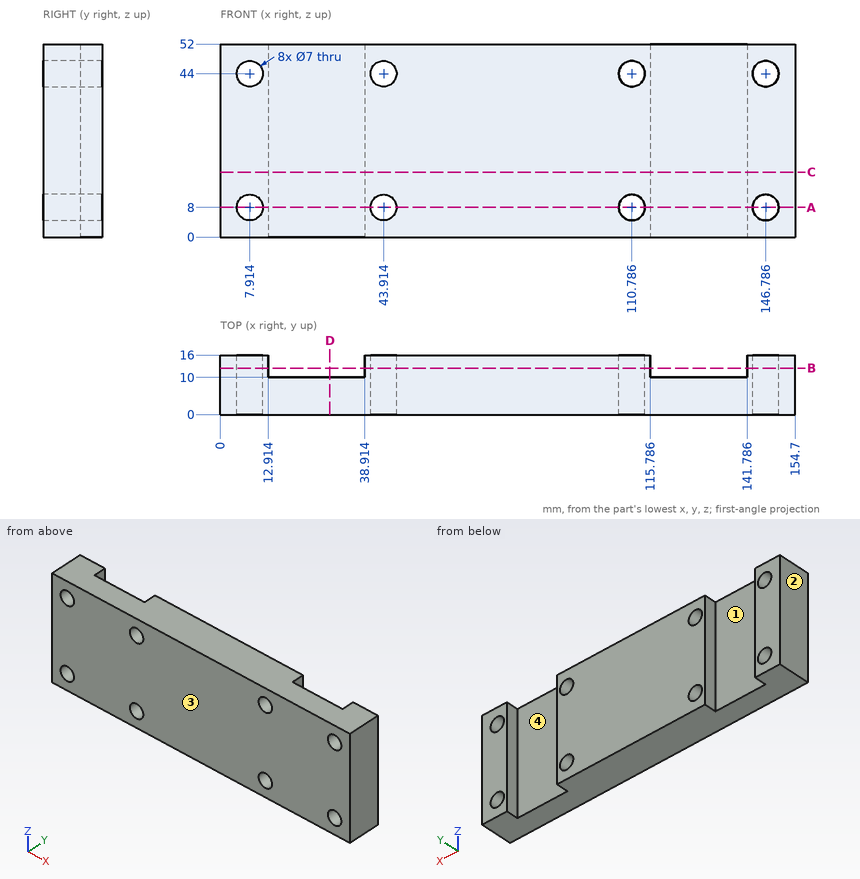
Here's the drawing with two shaded views (mm, measured from the low corner). I have some questions. Coordinates: 2 decimals unless noted, no trailing zeros. Order: outer loops, then holes, each group sorted by start corner. A loop starts at its lowest first (then second) coordinate and runs counter-clockwise, first axis right, second up. Notation, with made-up numbers: (46, -35.5) -> (102, -35.5) arc R19 cw to (102, -2.5) -> close; hole circle Ø10 at (42, 39.5). An arc over 180 degrees is marked (long way). Write each question's results on one line, items separated by ' | '.
Item 1: I want a section at D-D, the plane x = 29.5. Write out the boundary of the cut face in (y, z).
Results are:
outline: (0, 0) -> (10, 0) -> (10, 52) -> (0, 52) -> close
Item 2: If we mould it in two halves opening along X, with no side actions, what happens to the marked faces 1, 2, 3 and 4? For each: +X half, -X half, draft (parallel to the pull), parting line (faces both ways), or undercut.
Results are:
face 1: undercut | face 2: -X half | face 3: draft | face 4: undercut
Item 3: If I drill on line 1 along X through (y, z) = (7, 8) (1 decimal); line 2 along X through (y, z) = (11.25, 2) (1 decimal); line 3 along Z through (x, y) = (44, 7.75), over which ranges is the centre line in solid material (lowest first)?
Results are:
line 1: 0 to 4.4, 11.4 to 40.4, 47.4 to 107.3, 114.3 to 143.3, 150.3 to 154.7 | line 2: 0 to 12.9, 38.9 to 115.8, 141.8 to 154.7 | line 3: 0 to 4.5, 11.5 to 40.5, 47.5 to 52
Item 4: I want a section at A-A, the plane z = 8. Write out the boundary of the cut face in (x, y) (1 decimal).
Results are:
outline: (0, 0) -> (4.4, 0) -> (4.4, 16) -> (0, 16) -> close; (11.4, 0) -> (40.4, 0) -> (40.4, 16) -> (38.9, 16) -> (38.9, 10) -> (12.9, 10) -> (12.9, 16) -> (11.4, 16) -> close; (47.4, 0) -> (107.3, 0) -> (107.3, 16) -> (47.4, 16) -> close; (114.3, 0) -> (143.3, 0) -> (143.3, 16) -> (141.8, 16) -> (141.8, 10) -> (115.8, 10) -> (115.8, 16) -> (114.3, 16) -> close; (150.3, 0) -> (154.7, 0) -> (154.7, 16) -> (150.3, 16) -> close
Item 5: I want a section at C-C, the plane z = 17.5. Write out the boundary of the cut face in (x, y) (1 decimal), then the cut area to 3 significant figures.
Results are:
outline: (0, 0) -> (154.7, 0) -> (154.7, 16) -> (141.8, 16) -> (141.8, 10) -> (115.8, 10) -> (115.8, 16) -> (38.9, 16) -> (38.9, 10) -> (12.9, 10) -> (12.9, 16) -> (0, 16) -> close | area: 2,160 mm²
Item 6: I want a section at B-B, the plane y = 12.5. Count the separate pieces of the cut face and the enclosed holes in it, then the cut area to 3 significant figures.
Results are:
separate pieces: 3 | enclosed holes: 8 | area: 5,030 mm²
Item 7: I'm going to push flat-ended pins straight in: pin 1 Ø13 at (x, z) = (128, 33.5) entering from +Y; pin 2 Ø6.5 at (x, z) = (146.79, 8) entering from +Y. Where does each tip first touch, or does it pass through?
Results are:
pin 1: y = 10 | pin 2: through
